Source: CAD feature listing. Evaluate the final solid. Frame: model axes, mm. A direction names the side the tool comes from. Coordinates: 2 decimals unless noted, no trailing zeros. Write each loop counter-clockwise with the first axis right and the second up, starting at its lowest first coordinate (ties: lowest second). Pieces come first, ordered by that corner, then holes. Notation, with made-up numbers: (84.5, -9) - (116.5, -9) arc R31 cw to (116.5, 20) - close; hole circle Ø11 at (-15, 40). An arc over 180 degrees is marked (long way). One line per item, written item: value.
from build123d import *

# Parameters (mm, degrees)
F0_R         = 34.925
F1_DEPTH     = 50.8
F2_DEPTH     = 12.7
F0_R_2       = 12.7
F3_DEPTH     = 25.4
F4_F1_R      = 3.175
F4_F2_R      = 3.175
F4_F3_R      = 3.175
F4_F4_R      = 3.175
F4_F5_R      = 3.175
F4_T9_DEPTH  = 264.3151886434
F4_S10_R     = 27.051
F4_T11_DEPTH = 134
F4_S12_R     = 53.975
F4_T13_DEPTH = 134
F4_T17_DEPTH = 264.3151886434
F4_S18_R     = 27.051
F4_T19_DEPTH = 134
F4_S20_R     = 53.975
F4_T21_DEPTH = 134


# Not quite as in the source:
# - a fillet or chamfer that OpenCascade refuses, or shapes differently, is made with other operations: its cross-section is extruded or revolved along the edge and cut away or added


with BuildPart() as f1:
    # F0 (on Top) → F1 (new body)
    with BuildSketch(Plane.XY):
        with BuildLine():
            ThreePointArc((-174.625, 0), (-188.2488990323, 35.8481418723), (-222.2429444444, 53.5993327352))
            ThreePointArc((-222.2429444444, 53.5993327352), (-282.575, 0), (-222.2429444444, -53.5993327352))
            ThreePointArc((-222.2429444444, -53.5993327352), (-188.2488990323, -35.8481418723), (-174.625, 0))
        make_face()
        with Locations((-228.6, 0)):
            Circle(F0_R, mode=Mode.SUBTRACT)
    extrude(amount=F1_DEPTH)

    # F0 (on Top) → F2 (join)
    with BuildSketch(Plane.XY):
        with BuildLine():
            ThreePointArc((3.1860066667, -26.8627244061), (-27.051, 0), (3.1860066667, 26.8627244061))
            Line((3.1860066667, 26.8627244061), (-222.2429444444, 53.5993327352))
            ThreePointArc((-222.2429444444, 53.5993327352), (-188.2488990323, 35.8481418723), (-174.625, 0))
            ThreePointArc((-174.625, 0), (-188.2488990323, -35.8481418723), (-222.2429444444, -53.5993327352))
            Line((-222.2429444444, -53.5993327352), (3.1860066667, -26.8627244061))
        make_face()
        with BuildLine():
            ThreePointArc((-63.5, 15.875), (-52.2746798487, 11.2253201513), (-47.625, 0))
            ThreePointArc((-47.625, 0), (-52.2746798487, -11.2253201513), (-63.5, -15.875))
            Line((-63.5, -15.875), (-152.4, -15.875))
            ThreePointArc((-152.4, -15.875), (-168.275, 0), (-152.4, 15.875))
            Line((-152.4, 15.875), (-63.5, 15.875))
        make_face(mode=Mode.SUBTRACT)
    extrude(amount=F2_DEPTH)

    # F0 (on Top) → F3 (join)
    with BuildSketch(Plane.XY):
        with BuildLine():
            ThreePointArc((3.1860066667, -26.8627244061), (20.2230223673, -17.9662452207), (27.051, 0))
            ThreePointArc((27.051, 0), (20.2230223673, 17.9662452207), (3.1860066667, 26.8627244061))
            ThreePointArc((3.1860066667, 26.8627244061), (-27.051, 0), (3.1860066667, -26.8627244061))
        make_face()
        Circle(F0_R_2, mode=Mode.SUBTRACT)
    extrude(amount=F3_DEPTH)

    # F4: fillet of radius 3.175 on 10 edges, made by hand

    # F4_f1
    f4_f1_edges = [f1.edges().sort_by_distance(p)[0] for p in [
        (-234.9570555556, 53.5993327352, 50.8),
    ]]
    fillet(f4_f1_edges, radius=F4_F1_R)

    # F4_f2
    f4_f2_edges = [f1.edges().sort_by_distance(p)[0] for p in [
        (-47.625, 0, 12.7),
        (-107.95, -15.875, 12.7),
        (-168.275, 0, 12.7),
        (-107.95, 15.875, 12.7),
    ]]
    fillet(f4_f2_edges, radius=F4_F2_R)

    # F4_f3
    f4_f3_edges = [f1.edges().sort_by_distance(p)[0] for p in [
        (-263.525, 0, 50.8),
    ]]
    fillet(f4_f3_edges, radius=F4_F3_R)

    # F4_f4
    f4_f4_edges = [f1.edges().sort_by_distance(p)[0] for p in [
        (-3.1860066667, 26.8627244061, 25.4),
    ]]
    fillet(f4_f4_edges, radius=F4_F4_R)

    # F4_f5
    f4_f5_edges = [f1.edges().sort_by_distance(p)[0] for p in [
        (-12.7, 0, 25.4),
    ]]
    fillet(f4_f5_edges, radius=F4_F5_R)


with BuildPart() as f4_tool7:
    # F4_s8 → F4_t9 (new body)
    with BuildSketch(Plane(origin=(-249.0757155531, -29.5411916624, 0), x_dir=(0, 0, 1), z_dir=(0.9930399766, 0.1177777778, 0))):
        with BuildLine():
            ThreePointArc((12.7, 23.876), (11.7700640303, 26.1210640303), (9.525, 27.051))
            Line((9.525, 27.051), (9.525, 27.1145))
            Line((9.525, 27.1145), (12.7635, 27.1145))
            Line((12.7635, 27.1145), (12.7635, 23.876))
            Line((12.7635, 23.876), (12.7, 23.876))
        make_face()
    extrude(amount=F4_T9_DEPTH)

    # F4_s10 → F4_t11 (cut, symmetric)
    with BuildSketch(Plane.XY.offset(11.1)):
        Circle(F4_S10_R)
    extrude(amount=F4_T11_DEPTH, both=True, mode=Mode.SUBTRACT)

    # F4_s12 → F4_t13 (cut, symmetric)
    with BuildSketch(Plane.XY.offset(11.1)):
        with Locations((-228.6, 0)):
            Circle(F4_S12_R)
    extrude(amount=F4_T13_DEPTH, both=True, mode=Mode.SUBTRACT)


with BuildPart() as f1_1:
    add(f1.part)

    # F4_t6: cut F4_tool7
    add(f4_tool7.part, mode=Mode.SUBTRACT)


with BuildPart() as f4_tool15:
    # F4_s16 → F4_t17 (new body)
    with BuildSketch(Plane(origin=(13.3998331838, -1.5892638889, 0), x_dir=(0, 0, 1), z_dir=(-0.9930399766, 0.1177777778, 0))):
        with BuildLine():
            ThreePointArc((9.525, 27.051), (11.7700640303, 26.1210640303), (12.7, 23.876))
            Line((12.7, 23.876), (12.7635, 23.876))
            Line((12.7635, 23.876), (12.7635, 27.1145))
            Line((12.7635, 27.1145), (9.525, 27.1145))
            Line((9.525, 27.1145), (9.525, 27.051))
        make_face()
    extrude(amount=F4_T17_DEPTH)

    # F4_s18 → F4_t19 (cut, symmetric)
    with BuildSketch(Plane.XY.offset(11.1)):
        Circle(F4_S18_R)
    extrude(amount=F4_T19_DEPTH, both=True, mode=Mode.SUBTRACT)

    # F4_s20 → F4_t21 (cut, symmetric)
    with BuildSketch(Plane.XY.offset(11.1)):
        with Locations((-228.6, 0)):
            Circle(F4_S20_R)
    extrude(amount=F4_T21_DEPTH, both=True, mode=Mode.SUBTRACT)


with BuildPart() as f1_2:
    add(f1_1.part)

    # F4_t14: cut F4_tool15
    add(f4_tool15.part, mode=Mode.SUBTRACT)


solid = f1_2.part
1) Material intervals for line 1 (Y direction, x = -228, z = 34); line 2 (Y direction, x = 0, z = 17); line 3 (X direction, y = -24, z = 21.5), sorted ascending.
Values found:
line 1: -53.97 to -34.92, 34.92 to 53.97
line 2: -27.05 to -12.7, 12.7 to 27.05
line 3: -276.95 to -253.97, -203.23 to -180.25, -12.48 to 12.48
2) Section query B-B on y = 8. State how many separate pieces and enclosed holes the cut face has, then the cut area to 3 significant figures.
Values found:
separate pieces: 4
enclosed holes: 0
area: 3,180 mm2
3) Draft query along X for faces 4 (the flat face through (5, -16, 25.4)), 5 (the flat face through (-109, 22, 12.7)), 6 (the flat face through (-111.11, -40.42, 4.7)), 7 (the cylindrical face through (-195.288, 10.491, 23.479)). Return one class per face: released by +X, released by -X, zero draft, split by the parting line, or undercut.
Values found:
face 4: zero draft
face 5: undercut
face 6: released by +X
face 7: undercut
4) Contact query for flat-ended pins moving along their axis: P1, Ø1.5, axis at x = -186, z = 13.5, coming from the +Y side; P2, Ø3, axis at x = -118, z = 3, coming from the +Y side; P3, Ø10, axis at y = -18.5, z = 28, coming from the +X side; P4, Ø15, axis at x = 0, y = 0, coming from the -Z side. Output: stop coordinate, or through.
Values found:
P1: y = 34.09
P2: y = 41.41
P3: x = 21.51
P4: through
5) Section query A-A on z = 44.5. Output: boundary loops of the cut face in (x, y) (3 decimals), then the cut area to 3 significant figures.
Values found:
outline: circle Ø107.95 at (-228.6, 0); hole circle Ø69.85 at (-228.6, 0)
area: 5,320 mm2
6) Reachability of faces 1 (the cylindrical face through (-168.27, -0.35, 4.7)), 2 (the flat face through (-221, 38, 50.8)), 3 (the cylindrical face through (25.8, 8.13, 13.43)) from +Z, -Z, +X, -X, +Y, -Y: full face, straight path, thin tool, end or side. Return the list, or none.
Values found:
face 1: +Z, -Z
face 2: +Z, +X, -X, +Y, -Y
face 3: +Z
